Can you work these out from the model? Positions are in its coordinate system, mm. Face numbers are marked on the shaded views. A direction names the side the tool comes from. Coordinates: 2 decimals unless noted, no trailing zeros. Order: outer loops, then holes, each group sorted by start corner. A loop starts at its lowest first (then second) coordinate and runs counter-clockwise, first axis right, second up. Notation, with made-up numbers: (27, 26) -> (42, 26) arc R11 ccw to (42, 36) -> close; hole circle Ø9 at (-1, -37.5). An arc over 180 degrees is marked (long way). Answer in a Markdown table with one row per item.
```python
from build123d import *

# Parameters (mm, degrees)
SKETCH1_W           = 34
SKETCH1_H           = 24
SKETCH1_R           = 2.25
SKETCH1_W_2         = 22.6
SKETCH1_H_2         = 12
BOSS_EXTRUDE1_DEPTH = 3
FILLET1_R           = 0.5
FILLET2_R           = 2


with BuildPart() as part:
    # Sketch1 → Boss-Extrude1 (new body)
    with BuildSketch(Plane(origin=(0, 0, 0), x_dir=(1, 0, 0), z_dir=(0, 1, 0))):
        Rectangle(SKETCH1_W, SKETCH1_H)
        with Locations((-13.5, -9)):
            Circle(SKETCH1_R, mode=Mode.SUBTRACT)
        with Locations((-13.5, 9)):
            Circle(SKETCH1_R, mode=Mode.SUBTRACT)
        with Locations((13.5, -9)):
            Circle(SKETCH1_R, mode=Mode.SUBTRACT)
        with Locations((13.5, 9)):
            Circle(SKETCH1_R, mode=Mode.SUBTRACT)
        Rectangle(SKETCH1_W_2, SKETCH1_H_2, mode=Mode.SUBTRACT)
    extrude(amount=BOSS_EXTRUDE1_DEPTH)

    # Fillet1
    fillet1_edges = [part.edges().sort_by_distance(p)[0] for p in [
        (11.3, 1.5, 6),
        (11.3, 1.5, -6),
        (-11.3, 1.5, -6),
        (-11.3, 1.5, 6),
    ]]
    fillet(fillet1_edges, radius=FILLET1_R)

    # Fillet2
    fillet2_edges = [part.edges().sort_by_distance(p)[0] for p in [
        (17, 1.5, 12),
        (-17, 1.5, 12),
        (-17, 1.5, -12),
        (17, 1.5, -12),
    ]]
    fillet(fillet2_edges, radius=FILLET2_R)


solid = part.part
```
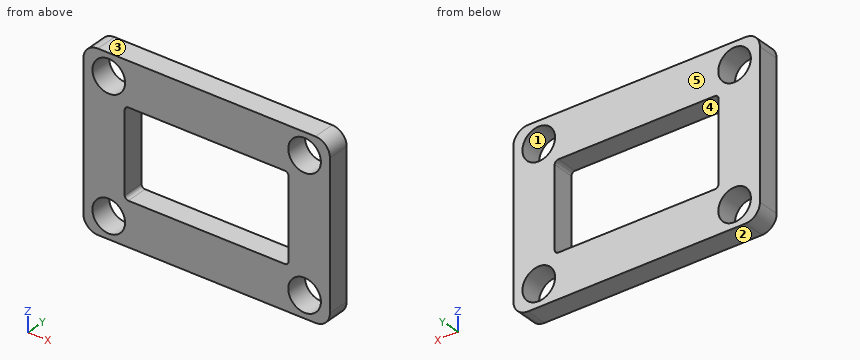
(1) On a 3-axis mill with a long thin cutter (end or side, diameter ignored), from which of +Z, -Z, +X, -X, +Y, -Y can I reach the whole of each face in a straight line? I mean the marked faces 4 and 5. Say none if no direction works.
Response values:
| item | result |
|---|---|
| face 4 | +Y, -Y |
| face 5 | +Z, -Z, +X, -X, +Y |
(2) Suppose I cut it at C-C (y = 0.65). Please give me the cut outline in (x, z).
Response values:
| item | result |
|---|---|
| outline | (-17, -10) arc R2 ccw to (-15, -12) -> (15, -12) arc R2 ccw to (17, -10) -> (17, 10) arc R2 ccw to (15, 12) -> (-15, 12) arc R2 ccw to (-17, 10) -> close; hole circle Ø4.5 at (-13.5, -9); hole circle Ø4.5 at (-13.5, 9); hole (-11.3, -5.5) arc R0.5 ccw to (-10.8, -6) -> (10.8, -6) arc R0.5 ccw to (11.3, -5.5) -> (11.3, 5.5) arc R0.5 ccw to (10.8, 6) -> (-10.8, 6) arc R0.5 ccw to (-11.3, 5.5) -> close; hole circle Ø4.5 at (13.5, -9); hole circle Ø4.5 at (13.5, 9) |
(3) We'd pull the mould along Z, two halves only. Please class the marked faces 1, 2 and 3: +Z half, -Z half, draft (parallel to the pull), parting line (faces both ways), or undercut.
Response values:
| item | result |
|---|---|
| face 1 | undercut |
| face 2 | -Z half |
| face 3 | +Z half |
(4) I need wall thicknesses on line 1 (Z direction, x = 13.5, y = 1.5); line 2 (X direction, y = 0.95, z = -9); line 3 (Z direction, x = -7.5, y = 0.1). Which ranges of each line are inside material? Lowest first, please. Write a range as [from, to].
Response values:
| item | result |
|---|---|
| line 1 | [-12, -11.25], [-6.75, 6.75], [11.25, 12] |
| line 2 | [-17, -15.75], [-11.25, 11.25], [15.75, 17] |
| line 3 | [-12, -6], [6, 12] |
(5) Suppose I cut it at D-D (z = -2). Please give me the cut outline in (x, y).
Response values:
| item | result |
|---|---|
| outline | (-17, 0) -> (-11.3, 0) -> (-11.3, 3) -> (-17, 3) -> close; (11.3, 0) -> (17, 0) -> (17, 3) -> (11.3, 3) -> close |
(6) Suppose I cut it at B-B (x = -2.5). Please give me the cut outline in (y, z), and give its area (3 significant figures).
Response values:
| item | result |
|---|---|
| outline | (0, -12) -> (3, -12) -> (3, -6) -> (0, -6) -> close; (0, 6) -> (3, 6) -> (3, 12) -> (0, 12) -> close |
| area | 36.0 mm2 |
(7) Suppose I cut it at A-A (z = -9). Please give me the cut outline in (x, y), and give its area (3 significant figures).
Response values:
| item | result |
|---|---|
| outline | (-17, 0) -> (-15.75, 0) -> (-15.75, 3) -> (-17, 3) -> close; (-11.25, 0) -> (11.25, 0) -> (11.25, 3) -> (-11.25, 3) -> close; (15.75, 0) -> (17, 0) -> (17, 3) -> (15.75, 3) -> close |
| area | 75.0 mm2 |
